from build123d import *

# Parameters (mm, degrees)
SKETCH1_R           = 50.3
BOSS_EXTRUDE1_DEPTH = 6.35
CUT_EXTRUDE1_REACH  = 85.65
SKETCH2_R           = 1.15
CIRPATTERN1_COUNT   = 3


with BuildPart() as part:
    # Sketch1 → Boss-Extrude1 (new body)
    with BuildSketch(Plane(origin=(0, 0, 0), x_dir=(1, 0, 0), z_dir=(0, 1, 0))):
        with BuildLine():
            Line((-10, -53.87986637), (-10, -62.87986637))
            Line((-10, -62.87986637), (10, -62.87986637))
            Line((10, -62.87986637), (10, -53.87986637))
            ThreePointArc((10, -53.87986637), (0, 54.8), (-10, -53.87986637))
        make_face()
        with Locations(Location((0, 0, 0), (0, 0, 270))):
            Circle(SKETCH1_R, mode=Mode.SUBTRACT)
    extrude(amount=BOSS_EXTRUDE1_DEPTH)

    # Sketch2 → Cut-Extrude1 (cut, up to next)
    with BuildSketch(Plane(origin=(0, 6.35, 0), x_dir=(1, 0, 0), z_dir=(0, 1, 0)), mode=Mode.PRIVATE) as cut_extrude1_sk1:
        with Locations(Location((0, -52.55, 0), (0, 0, 270))):
            Circle(SKETCH2_R)
    cut_extrude1_tool1 = extrude(cut_extrude1_sk1.sketch, amount=-CUT_EXTRUDE1_REACH, mode=Mode.PRIVATE) & part.part
    cut_extrude1 = cut_extrude1_tool1.solids().sort_by_distance((0, 6.35, 52.55))[0]
    add(cut_extrude1, mode=Mode.SUBTRACT)

    # CirPattern1: Cut-Extrude1 ×3 about axis
    cirpattern1_axis = Axis((0, 0, 0), (0, 1, 0))
    for i in range(1, CIRPATTERN1_COUNT):
        add(cut_extrude1.rotate(cirpattern1_axis, i * 360 / CIRPATTERN1_COUNT), mode=Mode.SUBTRACT)


solid = part.part
For this review, take the finished solid that the model builds, in its own axes (mm). Round coordinates to 2 decimals unless told otherwise and drop trailing zeros. Loops run counter-clockwise (first coordinate to the right, second up) from the corner with the lowest first, then second, coordinate; pieces in that order, holes last. Notation, with made-up numbers: (51, 85) - (70, 85) arc R32 cw to (70, 120) - close; hole circle Ø7 at (44.25, 13.25). An arc over 180 degrees is marked (long way). One line per question, with ' | ' between items.
Q1. The part is to be moulded in two halves that separate along X. For faces 1 (the flat face through (10, 3, 58)), 2 (the flat face through (-10, 3, 58)), 3 (the cylindrical face through (-30.607, 3.131, -39.916)), say which applies: released by +X, released by -X, zero draft, split by the parting line, or undercut.
Taken from the geometry:
face 1: released by +X | face 2: released by -X | face 3: undercut
Q2. Take a section at A-A (z = 0). Give the boundary of the cut face in (x, y), and give its area (4 significant figures).
Taken from the geometry:
outline: (-54.8, 0) - (-50.3, 0) - (-50.3, 6.35) - (-54.8, 6.35) - close; (50.3, 0) - (54.8, 0) - (54.8, 6.35) - (50.3, 6.35) - close | area: 57.15 mm²
Q3. Take a section at B-B (x = -8.5). Give the boundary of the cut face in (y, z).
Taken from the geometry:
outline: (0, -54.14) - (6.35, -54.14) - (6.35, -49.58) - (0, -49.58) - close; (0, 49.58) - (6.35, 49.58) - (6.35, 62.88) - (0, 62.88) - close
Q4. For pin 1 (3 mm diameter, centred on x = -45.51, z = -26.28, fed in from -Y); pin 2 (2 mm diameter, centred on x = 45.51, z = -26.27, fed in from -Y); pin 3 (1 mm diameter, centred on y = 5, z = 38.5, fed in from -X); pin 4 (1.9 mm diameter, centred on y = 4, z = 59, fed in from -X), all flat-tipped, find the tip position at first contact; note any pin that passes through.
Taken from the geometry:
pin 1: stops at y = 0 | pin 2: passes through | pin 3: stops at x = -39.48 | pin 4: stops at x = -10
Q5. For line 1 along Z through (x, y) = (-36, 5.5); line 2 along Z through (x, y) = (-1.5, 2.25); line 3 along X through (y, z) = (4.75, 20.5), list the stretches that pass through material, from the lowest coordinate up. Write a range as [from, to].
Taken from the geometry:
line 1: z = [-41.32, -35.13], [35.13, 41.32] | line 2: z = [-54.78, -50.28], [50.28, 62.88] | line 3: x = [-50.82, -45.93], [45.93, 50.82]
Q6. Take a section at C-C (y = 5.25). Give the boundary of the cut face in (x, z) (3 decimals), and give its area (3 significant figures).
Taken from the geometry:
outline: (-10, 53.88) arc R54.8 ccw (long way) to (10, 53.88) - (10, 62.88) - (-10, 62.88) - close; hole circle Ø100.6 at (0, 0); hole circle Ø2.3 at (-45.51, -26.275); hole circle Ø2.3 at (0, 52.55); hole circle Ø2.3 at (45.51, -26.275) | area: 1,640 mm²
